Could you check a few things on this model? Use its own coordinates, in mm. A direction names the side the tool comes from. Round coordinates to 2 decimals unless told otherwise and drop trailing zeros. Write each loop counter-clockwise with the first axis right and the second up, starting at its lowest first coordinate (ties: lowest second). Pieces come first, ordered by that corner, then holes. Notation, with made-up numbers: (63.5, 61) - (113.5, 61) arc R28 ccw to (113.5, 86) - close; hole circle Ø3 at (-0.5, 30.25). An arc over 180 degrees is marked (long way). Put each result on its own line as item: value.
from build123d import *

# Parameters (mm, degrees)
CUT_EXTRUDE1_DEPTH      = 60.252362822
CUT_EXTRUDE1_DEPTH_BACK = 60.252362822
SKETCH2_R               = 1
CUT_EXTRUDE2_DEPTH      = 60.252362859
CUT_EXTRUDE2_DEPTH_BACK = 60.252362859
SKETCH3_W               = 26
SKETCH3_H               = 3.2


with BuildPart() as part:
    # Sketch1 → Revolve1 (revolve)
    with BuildSketch(Plane.XY, mode=Mode.PRIVATE) as revolve1_sk:
        Polygon((-57.25, 0), (-57.25, 8), (-57.042201581, 8), (-48.45, 8), (-48.45, 5.8595471), (-48.45, 3.504470165), (-38.75, 3.504470165), (-38.75, 10.8), (-33.89, 10.8), (0, 10.8), (0, 10.3), (0.75, 10.3), (0.75, 10.8), (14.25, 10.8), (14.25, 0), align=None)
    revolve(revolve1_sk.sketch.rotate(Axis((-38.390119341, 0, 0), (1, 0, 0)), 90), axis=Axis((-38.390119341, 0, 0), (1, 0, 0)))

    # Sketch2 → Cut-Extrude1 (cut, two sides: drawn at the far end of the back side and taken through both)
    with BuildSketch(Plane.XY.offset(-CUT_EXTRUDE1_DEPTH_BACK)):
        with Locations((11.25, 0)):
            Circle(SKETCH2_R)
    extrude(amount=CUT_EXTRUDE1_DEPTH + CUT_EXTRUDE1_DEPTH_BACK, mode=Mode.SUBTRACT)

    # Sketch3 → Cut-Extrude2 (cut, two sides: drawn at the far end of the back side and taken through both)
    with BuildSketch(Plane(origin=(0, 0, 0), x_dir=(1, 0, 0), z_dir=(0, 1, 0)).offset(-CUT_EXTRUDE2_DEPTH_BACK)):
        with Locations((14.25, 0)):
            Rectangle(SKETCH3_W, SKETCH3_H)
    extrude(amount=CUT_EXTRUDE2_DEPTH + CUT_EXTRUDE2_DEPTH_BACK, mode=Mode.SUBTRACT)


solid = part.part
(1) For faces 1 (the face through (-52.91, 7.81, -1.73)), 2 (the face through (14.25, 0, 5)), 3 (the face through (10.46, -0.61, -6.26)), 4 (the face through (8, 0, 1.6)), 5 (the face through (-43.53, -2.37, -2.58)), which set-ups out of +Z, -Z, +X, -X, +Y, -Y let a thin tool reach every point of the face, with its end or its side?
Values found:
face 1: -X
face 2: +Z, -Z, +X, +Y, -Y
face 3: +Z, -Z
face 4: +X, +Y, -Y
face 5: none
(2) I'm going to push flat-ended pins straight in: pin 1 (3 mm diameter, centred on x = -9.5, y = 2, fed in from -Z); pin 2 (5 mm diameter, centred on x = -31.5, z = 3, fed in from +Y); pin 3 (1.5 mm diameter, centred on x = 4, y = -5.5, fed in from +Z). Where does each tip first touch, or does it pass through?
Values found:
pin 1: stops at z = -10.79
pin 2: stops at y = 10.79
pin 3: stops at z = 9.7
(3) Please list where these lines run through material, in increasing order: probe 1 along X at (y, z) = (-0.5, 4); probe 2 along Y at (x, z) = (-11, -1.5); probe 3 along X at (y, z) = (2, -4.5). Write a range as from..to.
Values found:
probe 1: x = -57.25..-48.45, -38.75..10.38, 12.12..14.25
probe 2: y = -10.7..10.7
probe 3: x = -57.25..-48.45, -38.75..14.25
(4) If we mould it in two halves opening along Z, with no side actions, what happens to faces 6 (the face through (7.594, 9.581, 4.984)), 7 (the face through (-38.75, -3, 3)), 8 (the face through (8, 0, -1.6)), 9 (the face through (1.25, 0, 0))? For each: pulls with the +Z half, pulls with the -Z half, needs draft (parallel to the pull), parting line crosses it, or undercut.
Values found:
face 6: parting line crosses it
face 7: needs draft
face 8: undercut
face 9: undercut
(5) Imagine slicing it at D-D, the plane z = 0. List the corners of the cut face in (x, y) for me, then the cut area to 3 significant figures.
Values found:
outline: (-57.25, -8) - (-48.45, -8) - (-48.45, -3.5) - (-38.75, -3.5) - (-38.75, -10.8) - (0, -10.8) - (0, -10.3) - (0.75, -10.3) - (0.75, -10.8) - (1.25, -10.8) - (1.25, 10.8) - (0.75, 10.8) - (0.75, 10.3) - (0, 10.3) - (0, 10.8) - (-38.75, 10.8) - (-38.75, 3.5) - (-48.45, 3.5) - (-48.45, 8) - (-57.25, 8) - close
area: 1,070 mm^2
(6) Imagine slicing it at A-A, the plane y = 0. Give the number of separate pieces and of enclosed holes in the cut face, then the cut area to 3 significant figures.
Values found:
separate pieces: 3
enclosed holes: 0
area: 1,270 mm^2
(7) Imagine slicing it at C-C, the plane x = 11.25. List the corners of the cut face in (y, z) for me, then the cut area to 3 significant figures.
Values found:
outline: (-10.68, -1.6) arc R10.8 ccw to (-1, -10.75) - (-1, -1.6) - close; (-10.68, 1.6) - (-1, 1.6) - (-1, 10.75) arc R10.8 ccw to start; (1, -10.75) arc R10.8 ccw to (10.68, -1.6) - (1, -1.6) - close; (1, 1.6) - (10.68, 1.6) arc R10.8 ccw to (1, 10.75) - close
area: 261 mm^2
(8) Imagine slicing it at B-B, the plane z = -4.5. List the corners of the cut face in (x, y) for me, then the cut area to 3 significant figures.
Values found:
outline: (-57.25, -6.61) - (-48.45, -6.61) - (-48.45, 6.61) - (-57.25, 6.61) - close; (-38.75, -9.82) - (0, -9.82) - (0, -9.26) - (0.75, -9.26) - (0.75, -9.82) - (14.25, -9.82) - (14.25, 9.82) - (0.75, 9.82) - (0.75, 9.26) - (0, 9.26) - (0, 9.82) - (-38.75, 9.82) - close; hole circle Ø2 at (11.25, 0)
area: 1,150 mm^2
